Here's how the part is built. I have some questions about the finished solid (model axes, mm). Round coordinates to 2 decimals unless told otherwise and drop trailing zeros. Order: outer loops, then holes, each group sorted by start corner. A loop starts at its lowest first (then second) coordinate and runs counter-clockwise, first axis right, second up. Notation, with made-up numbers: (-9, 78.5) - (21, 78.5) arc R22 cw to (21, 115.5) - close; hole circle Ø8 at (47, 73). An arc over 180 degrees is marked (long way). One line per item, written item: value.
from build123d import *

# Parameters (mm, degrees)
F0_W     = 63
F0_H     = 131
F0_W_2   = 131
F0_H_2   = 63
F0_W_3   = 62
F0_H_3   = 62
F1_DEPTH = 4
F0_W_4   = 4.3501859903
F0_H_4   = 22.087264806
F2_DEPTH = 4
F3_SIZE  = 3.99999
F4_DEPTH = 2


# Not quite as in the source:
# - a fillet or chamfer is up to 0.001 mm smaller than in the source, because OpenCascade refuses the exact size


with BuildPart() as f1:
    # F0 (on Top) → F1 (new body)
    with BuildSketch(Plane.XY):
        Polygon((110, 115.8440702578), (-110, 115.8440702578), (-110, -53.6358393729), (-105.6498140097, -53.6358393729), (-105.6498140097, -75.7231041789), (-110, -75.7231041789), (-110, -104.1559297422), (110, -104.1559297422), align=None)
        with Locations((-68.5, -28.6559297422)):
            Rectangle(F0_W, F0_H, mode=Mode.SUBTRACT)
        with Locations((34.5, -62.6559297422)):
            Rectangle(F0_W_2, F0_H_2, mode=Mode.SUBTRACT)
        with Locations((-34.5, 74.3440702578)):
            Rectangle(F0_W_2, F0_H_2, mode=Mode.SUBTRACT)
        with Locations((0, 5.8440702578)):
            Rectangle(F0_W_3, F0_H_3, mode=Mode.SUBTRACT)
        with Locations((68.5, 40.3440702578)):
            Rectangle(F0_W, F0_H, mode=Mode.SUBTRACT)
    extrude(amount=F1_DEPTH)

    # F0 (on Top) → F2 (join)
    with BuildSketch(Plane.XY):
        Polygon((110, 115.8440702578), (-110, 115.8440702578), (-110, -53.6358393729), (-105.6498140097, -53.6358393729), (-105.6498140097, -75.7231041789), (-110, -75.7231041789), (-110, -104.1559297422), (110, -104.1559297422), align=None)
        with Locations((-68.5, -28.6559297422)):
            Rectangle(F0_W, F0_H, mode=Mode.SUBTRACT)
        with Locations((34.5, -62.6559297422)):
            Rectangle(F0_W_2, F0_H_2, mode=Mode.SUBTRACT)
        with Locations((-34.5, 74.3440702578)):
            Rectangle(F0_W_2, F0_H_2, mode=Mode.SUBTRACT)
        with Locations((0, 5.8440702578)):
            Rectangle(F0_W_3, F0_H_3, mode=Mode.SUBTRACT)
        with Locations((68.5, 40.3440702578)):
            Rectangle(F0_W, F0_H, mode=Mode.SUBTRACT)
        with Locations((-107.8249070048, -64.6794717759)):
            Rectangle(F0_W_4, F0_H_4)
    extrude(amount=F2_DEPTH)

    # F3 (size 4 in the source; OpenCascade refuses exactly that, so slightly less here)
    f3_edges = [f1.edges().sort_by_distance(p)[0] for p in [
        (0, -104.15593, 4),
        (110, 5.84407, 4),
        (-110, 5.84407, 4),
        (0, 115.84407, 4),
    ]]
    chamfer(f3_edges, length=F3_SIZE)

    # F0 (on Top) → F4 (join)
    with BuildSketch(Plane.XY):
        with Locations((-107.8249070048, -64.6794717759)):
            Rectangle(F0_W_4, F0_H_4)
    extrude(amount=-F4_DEPTH)


solid = f1.part
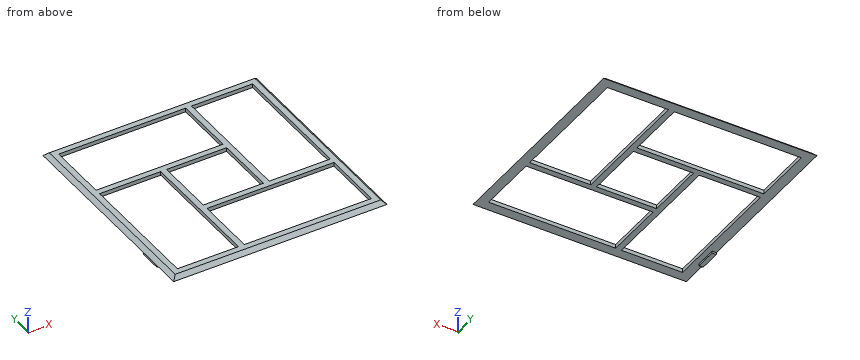
Q1. If we section it at D-D, the plane z = 1.65: Please give me the cut outline in (x, y), then the cut area to 3 significant figures.
Results list:
outline: (-108.35, -102.51) - (108.35, -102.51) - (108.35, 114.19) - (-108.35, 114.19) - close; hole (-100, -94.16) - (-37, -94.16) - (-37, 36.84) - (-100, 36.84) - close; hole (-100, 42.84) - (31, 42.84) - (31, 105.84) - (-100, 105.84) - close; hole (-31, -94.16) - (100, -94.16) - (100, -31.16) - (-31, -31.16) - close; hole (-31, -25.16) - (31, -25.16) - (31, 36.84) - (-31, 36.84) - close; hole (37, -25.16) - (100, -25.16) - (100, 105.84) - (37, 105.84) - close
area: 10,100 mm²
Q2. If I drill on line 1 along X through (y, z) = (-15, 2.9); line 2 along X through (y, z) = (70, 3.05); line 3 along X through (y, z) = (96.5, 1.95), over which ranges is the centre line in solid material (lowest first)?
Results list:
line 1: -107.1 to -100, -37 to -31, 31 to 37, 100 to 107.1
line 2: -106.95 to -100, 31 to 37, 100 to 106.95
line 3: -108.05 to -100, 31 to 37, 100 to 108.05
Q3. Will these pins go through, and if not, where does the flat tip stop? pin 1 (1.2 mm diameter, centred on y = 82, z = 1.5, fed in from +X); pin 2 (1.2 mm diameter, centred on x = 63.5, z = 2.5, fed in from -Y); pin 3 (1.2 mm diameter, centred on y = -43.5, z = 3, fed in from +X).
Results list:
pin 1: x = 109.1
pin 2: y = -102.26
pin 3: x = 107.6
Q4. If we section it at A-A, the plane x = -19: Give the number of separate pieces and of enclosed holes in the cut face, then the cut area to 3 significant figures.
Results list:
separate pieces: 4
enclosed holes: 0
area: 112 mm²
